For this review, take the finished solid that the model builds, in its own axes (mm). Give positions to 0.01 mm unless a question says otherwise; leave off trailing zeros. Write each loop counter-clockwise with the first axis right and the second up, starting at its lowest first coordinate (ties: lowest second). Pieces come first, ordered by that corner, then holes.
Q1. We need section D-D (x = -8). Write out the cut boundary in (y, z).
Q2. For line 1 (X direction, y = 1.15, z = -8) (3 decimals); line 2 (Z direction, x = 4.5, y = 1.05); line 3 (Z direction, x = -7.5, y = 0.5), list the stretches that pass through material, from the lowest coordinate up.
Q3. We need section C-C (x = 6.35). Give the number of separate pieces and of enclosed holes in the cut face, then the cut area to 3 significant figures.
Q4. We need section B-B (z = 8). Write out the cut boundary in (x, y).
```python
from build123d import *

# Parameters (mm, degrees)
SKETCH1_R           = 7
SKETCH1_R_2         = 2.25
BOSS_EXTRUDE1_DEPTH = 1.5875


with BuildPart() as part:
    # Sketch1 → Boss-Extrude1 (new body)
    with BuildSketch(Plane(origin=(0, 0, 0), x_dir=(1, 0, 0), z_dir=(0, 1, 0))):
        with BuildLine():
            Line((-15.875, 0), (-15.875, 30.1625))
            ThreePointArc((-15.875, 30.1625), (-15.410032015, 31.285032015), (-14.2875, 31.75))
            Line((-14.2875, 31.75), (14.2875, 31.75))
            ThreePointArc((14.2875, 31.75), (15.410032015, 31.285032015), (15.875, 30.1625))
            Line((15.875, 30.1625), (15.875, 0))
            ThreePointArc((15.875, 0), (0, -15.875), (-15.875, 0))
        make_face()
        Circle(SKETCH1_R, mode=Mode.SUBTRACT)
        with Locations((-8, 8)):
            Circle(SKETCH1_R_2, mode=Mode.SUBTRACT)
        with Locations((8, 8)):
            Circle(SKETCH1_R_2, mode=Mode.SUBTRACT)
        with Locations((8, -8)):
            Circle(SKETCH1_R_2, mode=Mode.SUBTRACT)
        with Locations((-8, -8)):
            Circle(SKETCH1_R_2, mode=Mode.SUBTRACT)
        with Locations((-6.35, 28.575)):
            Circle(SKETCH1_R_2, mode=Mode.SUBTRACT)
        with Locations((6.35, 15.875)):
            Circle(SKETCH1_R_2, mode=Mode.SUBTRACT)
    extrude(amount=BOSS_EXTRUDE1_DEPTH)


solid = part.part
```
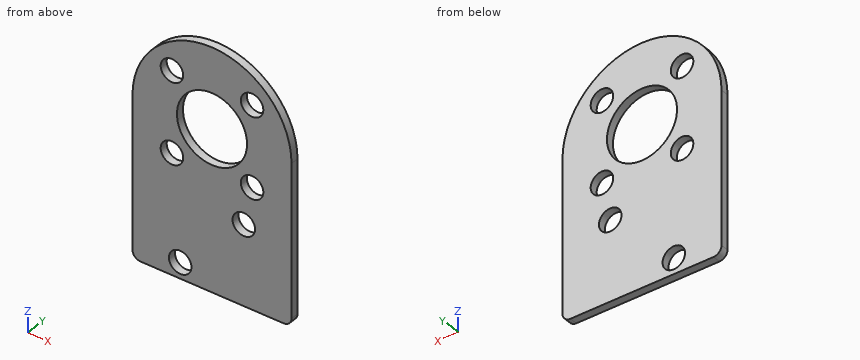
Computed:
1. outline: (0, -31.75) - (1.59, -31.75) - (1.59, -30.1) - (0, -30.1) - close; (0, -27.05) - (1.59, -27.05) - (1.59, -10.25) - (0, -10.25) - close; (0, -5.75) - (1.59, -5.75) - (1.59, 5.75) - (0, 5.75) - close; (0, 10.25) - (1.59, 10.25) - (1.59, 13.71) - (0, 13.71) - close
2. line 1: x = -15.875 to -10.25, -5.75 to 5.75, 10.25 to 15.875
2. line 2: z = -31.75 to -17.16, -14.59 to -5.36, 5.36 to 15.22
2. line 3: z = -31.75 to -30.51, -26.64 to -10.19, -5.81 to 5.81, 10.19 to 13.99
3. separate pieces: 5
3. enclosed holes: 0
3. area: 47.3 mm2
4. outline: (-13.71, 0) - (-10.25, 0) - (-10.25, 1.59) - (-13.71, 1.59) - close; (-5.75, 0) - (5.75, 0) - (5.75, 1.59) - (-5.75, 1.59) - close; (10.25, 0) - (13.71, 0) - (13.71, 1.59) - (10.25, 1.59) - close
